Geometry: final body of the model. Coordinates: model frame, mm. A direction names the side the tool comes from. Round coordinates to 2 decimals unless told otherwise and drop trailing zeros. Write each loop counter-clockwise with the first axis right and the second up, starting at its lowest first coordinate (ties: lowest second). Pieces come first, ordered by that corner, then holes. Notation, with made-up numbers: M 23,76.5 L 31,76.5 A8 cw 31,84.5 Z; hole C -18.5,-4.75 d11. An arc over 180 degrees is marked long. Answer as CSV lines item,"result". Start each with the question number.
Q1. Ray query, probe 1 along Y at (x, z) = (0, 5); probe 2 along Z at (x, y) = (-7, 3.5); probe 3 along Z at (x, y) = (1, -1.5). Return the intervals inside material, ascending.
Q2. Section query C-C on z = 19. Output: boundary loops of the cut face in (x, y), and give its area (3 significant figures).
Q3. Mould query, pull axis X, two halves, no side actions, for faces 1 (the flat face through (0, 0, 9)), 2 (the flat face through (5.2, 0.1, 31.9)), 3 (the cylindrical face through (2.337, -0.969, 4.437)), 4 (the cylindrical face through (-1.73, -7.81, 26.27)). Classes: pulls with the +X half, pulls with the -X half, needs draft (parallel to the pull), parting line crosses it, or undercut.
Q4. Section query D-D on z = 6. Output: boundary loops of the cut face in (x, y).
Q5. Section query A-A on x = 0. Output: boundary loops of the cut face in (y, z), and give its area (3 significant figures).
Q6. Reachability of faces 5 (the cylindrical face through (-1.08, -4.88, 42.75)), 6 (the flat face through (3, 0, 0)), 7 (the flat face through (-2, 6, 20.8)) from +Z, -Z, +X, -X, +Y, -Y: full face, straight path, thin tool, end or side. Return the list, or none.
Q7. First-contact query: pin 1 (4 mm diameter, centred on y = -2, z = 47.5, fed in from +X); pin 2 (1 mm diameter, centred on y = -0.5, z = 33.5, fed in from -X); pin 3 (4 mm diameter, centred on x = -4.5, z = 39, fed in from -Y). Flat tips, straight axial feed; report the tip coordinate or a pass-through.
```python
from build123d import *

# Parameters (mm, degrees)
S01_12_MM_BEARING_JOURNAL_R                  = 6
F_01_12_MM_BEARING_JOURNAL_DEPTH             = 20.8
F_02_START                                   = 20.8
S02_GROUNDED_JOURNAL_SHOULDER_R              = 8
F_02_GROUNDED_JOURNAL_SHOULDER_DEPTH         = 11.1
F_03_START                                   = 31.9
S03_M10_THREADED_BRIDGE_STEM_R               = 5
F_03_M10_THREADED_BRIDGE_STEM_DEPTH          = 22
F_04_START                                   = -0.1
S04_M5_TAPPED_END_NOMINAL_THREAD_ENV_R       = 2.53
F_04_M5_TAPPED_END_NOMINAL_THREAD_ENVE_DEPTH = 9.1


with BuildPart() as part:
    # S01 - 12 mm bearing journal → 01 - 12 mm bearing journal (new body)
    with BuildSketch(Plane.XY):
        Circle(S01_12_MM_BEARING_JOURNAL_R)
    extrude(amount=F_01_12_MM_BEARING_JOURNAL_DEPTH)

    # S02 - Grounded journal shoulder → 02 - Grounded journal shoulder (add)
    with BuildSketch(Plane.XY.offset(F_02_START)):
        Circle(S02_GROUNDED_JOURNAL_SHOULDER_R)
    extrude(amount=F_02_GROUNDED_JOURNAL_SHOULDER_DEPTH)

    # S03 - M10 threaded bridge stem → 03 - M10 threaded bridge stem (add)
    with BuildSketch(Plane.XY.offset(F_03_START)):
        Circle(S03_M10_THREADED_BRIDGE_STEM_R)
    extrude(amount=F_03_M10_THREADED_BRIDGE_STEM_DEPTH)

    # S04 - M5 tapped end - nominal thread envelope → 04 - M5 tapped end - nominal thread envelope (cut)
    with BuildSketch(Plane.XY.offset(F_04_START)):
        Circle(S04_M5_TAPPED_END_NOMINAL_THREAD_ENV_R)
    extrude(amount=F_04_M5_TAPPED_END_NOMINAL_THREAD_ENVE_DEPTH, mode=Mode.SUBTRACT)


solid = part.part
```
Entries:
1,probe 1,"y = -6 to -2.53, 2.53 to 6"
1,probe 2,"z = 20.8 to 31.9"
1,probe 3,"z = 9 to 53.9"
2,outline,"C 0,0 d12"
2,area,"113 mm^2"
3,face 1,"undercut"
3,face 2,"needs draft"
3,face 3,"undercut"
3,face 4,"parting line crosses it"
4,outline,"C 0,0 d12; hole C 0,0 d5.06"
5,outline,"M -8,20.8 L -6,20.8 L -6,0 L -2.53,0 L -2.53,9 L 2.53,9 L 2.53,0 L 6,0 L 6,20.8 L 8,20.8 L 8,31.9 L 5,31.9 L 5,53.9 L -5,53.9 L -5,31.9 L -8,31.9 Z"
5,area,"602 mm^2"
6,face 5,"+Z"
6,face 6,"-Z, +X, -X, +Y, -Y"
6,face 7,"-Z"
7,pin 1,"stops at x = 5"
7,pin 2,"stops at x = -5"
7,pin 3,"stops at y = -4.33"
